from build123d import *

# Parameters (mm, degrees)
ESQUISSE1_W                                    = 200
ESQUISSE1_H                                    = 100
BOSS_EXTRU_1_DEPTH                             = 10
FRAISAGE_POUR_VIS_T_TE_FRAIS_E_M61_D           = 6.2
FRAISAGE_POUR_VIS_T_TE_FRAIS_E_M61_CSINK_D     = 12.6
FRAISAGE_POUR_VIS_T_TE_FRAIS_E_M61_CSINK_ANGLE = 90


with BuildPart() as part:
    # Esquisse1 → Boss.-Extru.1 (new body)
    with BuildSketch(Plane(origin=(0, 0, 0), x_dir=(1, 0, 0), z_dir=(0, 1, 0))):
        Rectangle(ESQUISSE1_W, ESQUISSE1_H)
    extrude(amount=BOSS_EXTRU_1_DEPTH)

    # Fraisage pour vis à tête fraisée M61 (through all)
    with Locations(Plane(origin=(0, 0, 0), x_dir=(-1, 0, 0), z_dir=(0, -1, 0))):
        with Locations((-80, 20), (-80, -20)):
            CounterSinkHole(FRAISAGE_POUR_VIS_T_TE_FRAIS_E_M61_D / 2, FRAISAGE_POUR_VIS_T_TE_FRAIS_E_M61_CSINK_D / 2, counter_sink_angle=FRAISAGE_POUR_VIS_T_TE_FRAIS_E_M61_CSINK_ANGLE)


solid = part.part
Could you check a few things on this model? Use its own coordinates, in mm. Give positions to 0.01 mm unless a question says otherwise; leave off trailing zeros. Write each loop counter-clockwise with the first axis right and the second up, starting at its lowest first coordinate (ties: lowest second). Pieces come first, ordered by that corner, then holes. Notation, with made-up numbers: (-7, 3) - (17, 3) arc R10 cw to (17, 19) - close; hole circle Ø11 at (27, -8.75). An arc over 180 degrees is marked (long way). Use CSV: the item, a comma, the result in double quotes. Start each with the question number.
Item 1: If we mould it in two halves opening along X, with no side actions, what happens to faces 1 (the face through (100, 5, 1)), 2 (the face through (82.957, 6.648, 19.069)), 3 (the face through (-1, 0, -1))? For each: pulls with the +X half, pulls with the -X half, needs draft (parallel to the pull), parting line crosses it, or undercut.
Item 2: I want a section at B-B, the plane z = 20. Please give me the cut outline in (x, y).
Item 3: If I drill on line 1 along Z through (x, y) = (80, 6.5); line 2 along X through (y, z) = (6.75, -20); line 3 along X through (y, z) = (4.5, -19), over which ranges is the centre line in solid material (lowest first)?
Item 4: I want a section at A-A, the plane x = 80. Please give me the cut outline in (y, z), then the cut area to 3 significant figures.
Item 5: I'm going to push a flat-ended pin straight in: pin 1 (5.5 mm diameter, centred on x = 80, z = -20, fed in from +Y). Where does the tip first touch, or does it pass through?
Findings:
1,face 1,"pulls with the +X half"
1,face 2,"undercut"
1,face 3,"needs draft"
2,outline,"(-100, 0) - (73.7, 0) - (76.9, 3.2) - (76.9, 10) - (-100, 10) - close; (83.1, 3.2) - (86.3, 0) - (100, 0) - (100, 10) - (83.1, 10) - close"
3,line 1,"z = -50 to -23.1, -16.9 to 16.9, 23.1 to 50"
3,line 2,"x = -100 to 76.9, 83.1 to 100"
3,line 3,"x = -100 to 77.07, 82.93 to 100"
4,outline,"(0, -50) - (10, -50) - (10, -23.1) - (3.2, -23.1) - (0, -26.3) - close; (0, -13.7) - (3.2, -16.9) - (10, -16.9) - (10, 16.9) - (3.2, 16.9) - (0, 13.7) - close; (0, 26.3) - (3.2, 23.1) - (10, 23.1) - (10, 50) - (0, 50) - close"
4,area,"856 mm2"
5,pin 1,"passes through"
